from build123d import *

# Parameters (mm, degrees)
AUFSATZ_LINEAR_AUSTRAGEN2_DEPTH = 2
SKIZZE4_W                       = 30
SKIZZE4_H                       = 70
SKIZZE4_W_2                     = 26
SKIZZE4_H_2                     = 2.2
SCHNITT_LINEAR_AUSTRAGEN1_DEPTH = 2


with BuildPart() as part:
    # Skizze3 → Aufsatz-Linear austragen2 (new body)
    with BuildSketch(Plane(origin=(0, 0, 0), x_dir=(1, 0, 0), z_dir=(0, 1, 0))):
        Polygon((-29.8, 0), (0, 0), (0, 6), (10.85, 6), (10.85, 23.4), (14.85, 23.4), (14.85, 42.4), (10.85, 42.4), (10.85, 73.4), (14.85, 73.4), (14.85, 92.4), (10.85, 92.4), (10.85, 108.4), (0.1, 108.4), (0.1, 113.4), (-29.9, 113.4), (-29.9, 108.4), (-40.65, 108.4), (-40.65, 92.4), (-44.65, 92.4), (-44.65, 73.4), (-40.65, 73.4), (-40.65, 42.4), (-44.65, 42.4), (-44.65, 23.4), (-40.65, 23.4), (-40.65, 6), (-29.8, 6), align=None)
    extrude(amount=AUFSATZ_LINEAR_AUSTRAGEN2_DEPTH)

    # Skizze4 → Schnitt-Linear austragen1 (cut)
    with BuildSketch(Plane(origin=(0, 2, 0), x_dir=(1, 0, 0), z_dir=(0, 1, 0))):
        with Locations((-14.9, 57.449848024)):
            Rectangle(SKIZZE4_W, SKIZZE4_H)
        with Locations((-14.9, 2.9)):
            Rectangle(SKIZZE4_W_2, SKIZZE4_H_2)
    extrude(amount=-SCHNITT_LINEAR_AUSTRAGEN1_DEPTH, mode=Mode.SUBTRACT)


solid = part.part
Model file for the job. Use its own axes, mm. A direction names the side the tool comes from. Give positions to 0.01 mm unless a question says otherwise; leave off trailing zeros. Loops run counter-clockwise (first coordinate to the right, second up) from the corner with the lowest first, then second, coordinate; pieces in that order, holes last.
Item 1: Slice it at B-B (x = -19). Write the cut outline in (y, z), plus the area to 3 significant figures.
Check values:
outline: (0, -113.4) - (2, -113.4) - (2, -92.45) - (0, -92.45) - close; (0, -22.45) - (2, -22.45) - (2, -4) - (0, -4) - close; (0, -1.8) - (2, -1.8) - (2, 0) - (0, 0) - close
area: 82.4 mm2
Item 2: Drop flat-ended pins along their axis: P1, Ø0.6, axis at x = -43, y = 1, coming from the +Z side; P2, Ø1, axis at y = 1.5, z = -57.5, coming from the +X side; P3, Ø1.5, axis at x = 0.5, z = -65, coming from the -Y side; P4, Ø6, axis at x = -3, z = -41, coming from the +Y side. Give the stop position or say it passes through.
Check values:
P1: stops at z = -23.4
P2: stops at x = 10.85
P3: stops at y = 0
P4: passes through
Item 3: Mould opens along Z. For faces 1 (the face through (14.85, 1, -83)), 2 (the face through (-43, 1, -73.4)), 3 (the face through (5, 1, -6)) say: +Z half, -Z half, draft (parallel to the pull), parting line (faces both ways), or undercut.
Check values:
face 1: draft
face 2: undercut
face 3: +Z half
Item 4: Slice it at A-A (z = -74.5). Write the cut outline in (x, y).
Check values:
outline: (-44.65, 0) - (-29.9, 0) - (-29.9, 2) - (-44.65, 2) - close; (0.1, 0) - (14.85, 0) - (14.85, 2) - (0.1, 2) - close
Item 5: Slice it at C-C (z = -56.5). Write the cut outline in (x, y).
Check values:
outline: (-40.65, 0) - (-29.9, 0) - (-29.9, 2) - (-40.65, 2) - close; (0.1, 0) - (10.85, 0) - (10.85, 2) - (0.1, 2) - close
Item 6: Drill centre lines: line 1 along Z through (x, y) = (-10.5, 0.9); line 2 along X through (y, z) = (0.9, -82.5); line 3 along X through (y, z) = (1.3, -73). Where is each one in solid material? Low to high.
Check values:
line 1: z = -113.4 to -92.45, -22.45 to -4, -1.8 to 0
line 2: x = -44.65 to -29.9, 0.1 to 14.85
line 3: x = -40.65 to -29.9, 0.1 to 10.85
Item 7: Slice it at D-D (y = 0.85). Give the number of separate pieces and of enclosed holes in the cut face, plus the area to 3 significant figures.
Check values:
separate pieces: 1
enclosed holes: 2
area: 3,750 mm2
Item 8: Which spindle directions (+Z, -Z, +X, -X, +Y, -Y) get a long thin tool onto all of the face, cutting with end or side? Do faces 4 (the face through (10.85, 1, -15)), 5 (the face through (6, 1, -108.4)), 6 (the face through (-40.65, 1, -101)), 7 (the face through (-1.9, 1, -3)), 8 (the face through (-43, 1, -42.4)). Say none if no direction does.
Check values:
face 4: +Z, +X, +Y, -Y
face 5: -Z, +X, +Y, -Y
face 6: -Z, -X, +Y, -Y
face 7: +Y, -Y
face 8: -X, +Y, -Y
